from build123d import *

# Parameters (mm, degrees)
BOSS_EXTRUDE1_DEPTH = 23.8125
SKETCH2_R           = 3.5687
CUT_EXTRUDE1_DEPTH  = 26.4
SKETCH3_R           = 3.5687
CUT_EXTRUDE2_DEPTH  = 26.4


with BuildPart() as part:
    # Sketch1 → Boss-Extrude1 (new body, symmetric)
    with BuildSketch(Plane.XY):
        with BuildLine():
            Line((0, 0), (0, 25.4))
            ThreePointArc((0, 25.4), (3.376576302, 24.001376302), (4.7752, 20.6248))
            Line((4.7752, 20.6248), (4.7752, 7.9502))
            ThreePointArc((4.7752, 7.9502), (5.70513597, 5.70513597), (7.9502, 4.7752))
            Line((7.9502, 4.7752), (20.6248, 4.7752))
            ThreePointArc((20.6248, 4.7752), (24.001376302, 3.376576302), (25.4, 0))
            Line((25.4, 0), (0, 0))
        make_face()
    extrude(amount=BOSS_EXTRUDE1_DEPTH, both=True)

    # Sketch2 → Cut-Extrude1 (cut, through all)
    with BuildSketch(Plane(origin=(0, 0, 0), x_dir=(1, 0, 0), z_dir=(0, 1, 0))):
        with Locations((12.7, -12.7)):
            Circle(SKETCH2_R)
        with Locations((12.7, 12.7)):
            Circle(SKETCH2_R)
    extrude(amount=CUT_EXTRUDE1_DEPTH, mode=Mode.SUBTRACT)

    # Sketch3 → Cut-Extrude2 (cut, through all)
    with BuildSketch(Plane(origin=(0, 0, 0), x_dir=(0, 0, -1), z_dir=(1, 0, 0))):
        with Locations((-12.7, 12.7)):
            Circle(SKETCH3_R)
        with Locations((12.7, 12.7)):
            Circle(SKETCH3_R)
    extrude(amount=CUT_EXTRUDE2_DEPTH, mode=Mode.SUBTRACT)


solid = part.part
Geometry: final body of the model. Coordinates: model frame, mm. A direction names the side the tool comes from. Coordinates: 2 decimals unless noted, no trailing zeros. Loops run counter-clockwise (first coordinate to the right, second up) from the corner with the lowest first, then second, coordinate; pieces in that order, holes last. Notation, with made-up numbers: (89.25, -4) - (137.25, -4) arc R18 ccw to (137.25, 24) - close; hole circle Ø9 at (-29.75, 21.5). An arc over 180 degrees is marked (long way). Put each result on its own line as item: value. Start each with the question number.
Q1. Cut plane D-D, the plane z = 20.5. Return loops of the section in (x, y) (3 decimals), and give its area (3 significant figures).
Q2. Cut plane A-A, the plane y = 12.7. Return loops of the section in (x, z), and give its area (3 significant figures).
Q3. Pull-direction query (Y, two-part tool) for faces 1 (the flat face through (0, 13, 0)), 2 (the cylindrical face through (5.68, 5.73, 0.33)), 3 (the cylindrical face through (2.354, 9.216, 13.474)); classes: released by +Y, released by -Y, zero draft, split by the parting line, or undercut.
Q4. Set-up query: faces 4 (the flat face through (14, 4.775, 0)), 5 (the flat face through (7, 4, 23.812)). Return all of +Z, -Z, +X, -X, +Y, -Y with unobstructed straight access to the full face (end or side cutting, diameter ignored); none if empty.
Q5. Cut plane C-C, the plane z = -12.7. Return loops of the section in (x, y) (3 decimals).
Q6. Line query: line 1 (Z direction, x = 12.7, y = 1.1); line 2 (Y direction, x = 11, z = -1.5). Output: solid intervals per line, ascending.
Q7. Pin query (flat end, axial travel): pin 1 Ø6.5 at (y, z) = (12.7, 12.7) entering from +X; pin 2 Ø6 at (y, z) = (9, -6) entering from +X; pin 3 Ø10 at (x, z) = (5.5, 1.5) entering from +Y; pin 4 Ø14 at (y, z) = (16.5, 3.5) entering from +X. Return the tip coordinate at first contact, or that it passes through.
Filled sheet:
1. outline: (0, 0) - (25.4, 0) arc R4.775 ccw to (20.625, 4.775) - (7.95, 4.775) arc R3.175 cw to (4.775, 7.95) - (4.775, 20.625) arc R4.775 ccw to (0, 25.4) - close
1. area: 212 mm²
2. outline: (0, -23.81) - (4.78, -23.81) - (4.78, -16.27) - (0, -16.27) - close; (0, -9.13) - (4.78, -9.13) - (4.78, 9.13) - (0, 9.13) - close; (0, 16.27) - (4.78, 16.27) - (4.78, 23.81) - (0, 23.81) - close
2. area: 159 mm²
3. face 1: zero draft
3. face 2: released by +Y
3. face 3: undercut
4. face 4: +Z, -Z, +X, +Y
4. face 5: +Z, +X, -X, +Y, -Y
5. outline: (0, 0) - (9.131, 0) - (9.131, 4.775) - (7.95, 4.775) arc R3.175 cw to (4.775, 7.95) - (4.775, 9.131) - (0, 9.131) - close; (0, 16.269) - (4.775, 16.269) - (4.775, 20.625) arc R4.775 ccw to (0, 25.4) - close; (16.269, 0) - (25.4, 0) arc R4.775 ccw to (20.625, 4.775) - (16.269, 4.775) - close
6. line 1: -23.81 to -16.27, -9.13 to 9.13, 16.27 to 23.81
6. line 2: 0 to 4.78
7. pin 1: through
7. pin 2: x = 5.44
7. pin 3: y = 25.37
7. pin 4: x = 4.78
